Autodesk Inventor part; units mm, degrees
ref_plane "YZ Plane" through (0, 0, 0) normal (1, 0, 0) x (0, 1, 0)
ref_plane "XZ Plane" through (0, 0, 0) normal (0, 1, 0) x (-1, 0, 0)
ref_plane "XY Plane" through (0, 0, 0) normal (0, 0, 1) x (1, 0, 0)
sketch "Sketch1" plane through (0, 0, 0) normal (0, 1, 0) x (-1, 0, 0)
  line L0 (0, 0) -> (15, 0)
  line L1 (15, 0) -> (15, -33)
  line L2 (15, -33) -> (0, -33)
  line L3 (0, -33) -> (0, 0)
  dimension "d0" = 15
  dimension "d1" = 33
extrude "Extrusion1" add sketch "Sketch1" along normal blind 10
fillet "Fillet1" radius 2 2 edges at (0, 0, -16.5) (-15, 0, -16.5)
fillet "Fillet2" radius 2 10 edges at (-0.5858, 0.5858, -33) (-7.5, 0, -33) (-14.4142, 0.5858, -33) (-15, 6, -33) (0, 6, -33) (-0.5858, 0.5858, 0) (-7.5, 0, 0) (-14.4142, 0.5858, 0) (-15, 6, 0) (0, 6, 0)
sketch "Sketch2" plane through (0, 10, 0) normal (0, 1, 0) x (1, 0, 0)
  line L0 (-14.5243, 2) -> (-14.5243, 30.9154) construction
  line L1 (-14.5243, 30.9154) -> (-0.4504, 30.9154) construction
  line L2 (-0.4504, 30.9154) -> (-0.4504, 2) construction
  line L3 (-0.4504, 2) -> (-14.5243, 2) construction
properties material "ABS Plastic"
Input: part model. Units: mm. Frame: model coordinates. Coordinates: 2 decimals unless noted, no trailing zeros. Loops run counter-clockwise (first coordinate to the right, second up) from the corner with the lowest first, then second, coordinate; pieces in that order, holes last.
(1) Material intervals for probe 1 along Y at (x, z) = (-13.25, -7); probe 2 along X at (y, z) = (1, -28.5); probe 3 along Z at (x, y) = (-8.25, 1.75), sorted ascending.
(2) Section B-B on x = -13.5. Return the cut outline in (y, z), then the cut area to 3 significant figures.
(3) First-contact query: pin 1 Ø1 at (y, z) = (1.5, -22) entering from +X. Flat tip, straight axial feed; report the tip coordinate or a pass-through.
(4) Section A-A on y = 1. Return the cut outline in (x, z).
Data:
1. probe 1: y = 0.02 to 10
1. probe 2: x = -14.73 to -0.27
1. probe 3: z = -32.98 to -0.02
2. outline: (0.06, -31) arc R1.94 ccw to (2, -32.94) - (10, -32.94) - (10, -0.06) - (2, -0.06) arc R1.94 ccw to (0.06, -2) - close
2. area: 325 mm2
3. pin 1: stops at x = 0
4. outline: (-14.73, -31) arc R1.73 ccw to (-13, -32.73) - (-2, -32.73) arc R1.73 ccw to (-0.27, -31) - (-0.27, -2) arc R1.73 ccw to (-2, -0.27) - (-13, -0.27) arc R1.73 ccw to (-14.73, -2) - close
